```python
from build123d import *

# Parameters (mm, degrees)
SKETCH_1_W          = 8
SKETCH_1_H          = 29.75
SKETCH_1_R          = 1.5
EXTRUDE_1_DEPTH     = 1.5
SKETCH_2_W          = 2
SKETCH_2_H          = 8
EXTRUDE_2_DEPTH     = 16.5
FILLET_1_R          = 1
FILLET_2_R          = 1
SKETCH_4_R          = 1.5
CUT_EXTRUDE_1_DEPTH = 2


with BuildPart() as part:
    # 草图1 → 凸台-拉伸1 (new body)
    with BuildSketch(Plane.XY):
        Rectangle(SKETCH_1_W, SKETCH_1_H)
        with Locations((0, 11.875)):
            Circle(SKETCH_1_R, mode=Mode.SUBTRACT)
        with Locations((0, -11.875)):
            Circle(SKETCH_1_R, mode=Mode.SUBTRACT)
    extrude(amount=EXTRUDE_1_DEPTH)

    # 草图2 → 凸台-拉伸2 (add)
    with BuildSketch(Plane.XY.offset(1.5)):
        with Locations((0, 5)):
            Rectangle(SKETCH_2_W, SKETCH_2_H)
    extrude(amount=EXTRUDE_2_DEPTH)

    # 圆角1
    fillet_1_edges = [part.edges().sort_by_distance(p)[0] for p in [
        (1, 5, 1.5),
        (-1, 5, 1.5),
    ]]
    fillet(fillet_1_edges, radius=FILLET_1_R)

    # 圆角2
    fillet_2_edges = [part.edges().sort_by_distance(p)[0] for p in [
        (0, 9, 18),
        (0, 1, 18),
        (4, -14.875, 0.75),
        (-4, -14.875, 0.75),
        (-4, 14.875, 0.75),
        (4, 14.875, 0.75),
    ]]
    fillet(fillet_2_edges, radius=FILLET_2_R)

    # 草图4 → 切除-拉伸1 (cut)
    with BuildSketch(Plane.ZY.offset(1)):
        with Locations((14, 5)):
            Circle(SKETCH_4_R)
    extrude(amount=-CUT_EXTRUDE_1_DEPTH, mode=Mode.SUBTRACT)


solid = part.part
```
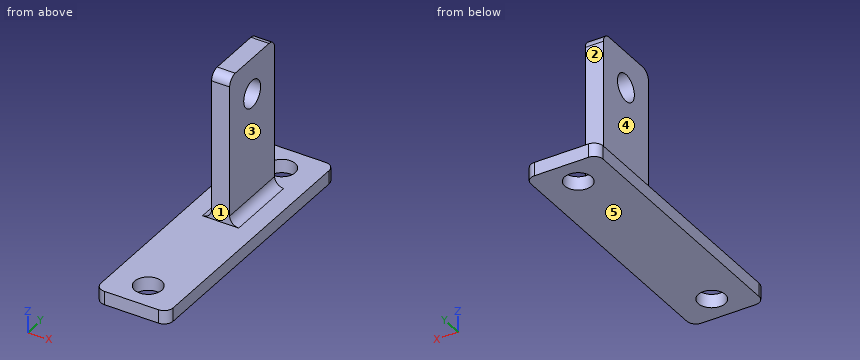
Verification items for the finished model (mm, model axes). Face numbers are marked on the shaded views. A direction names the side the tool comes from. Coordinates: 2 decimals unless noted, no trailing zeros. Write each loop counter-clockwise with the first axis right and the second up, starting at its lowest first coordinate (ties: lowest second). Pieces come first, ordered by that corner, then holes. Notation, with made-up numbers: (14.5, -2) - (72.5, -2) arc R13 cw to (72.5, 8) - close; hole circle Ø11 at (10.5, -14.75). An arc over 180 degrees is marked (long way). One line per question, with ' | ' between items. Start each with the question number.
1. Material ranges on line 1 along Y through (x, z) = (0, 1.25) (3 decimals); line 2 along Y through (x, z) = (-0.25, 14); line 3 along Z through (x, y) = (2, 9.5), recorded low to high.
2. Section check D-D (x = -2.5). Enter the section's corners in (y, z) (3 decimals).
3. Gauge pin test, flat ends, axial feed: P1, Ø8, axis at y = 0, z = 13, coming from the -X side; P2, Ø1.8, axis at x = 0, y = -11.875, coming from the -Z side; P3, Ø1.2, axis at x = 0.5, z = 10, coming from the -Y side; P4, Ø3, axis at x = -0.5, y = -5.5, coming from the +Z side. Record the tip position at first contact, or that the pin passes through.
4. Section check A-A (y = 5). Enter the section's corners in (x, z), plus the area to 3 significant figures.
5. Access from +Z, -Z, +X, -X, +Y, -Y to the whole of each face (thin tool, end or side, straight path). Record for the marked faces 1, 2, 3, 4 and 5.
6. Section check C-C (z = 14). Enter the section's corners in (x, y).
7. Section check B-B (x = 0). Enter the section's corners in (y, z) (3 decimals), plus the area to 3 significant figures.
Computed values:
1) line 1: -14.875 to -13.375, -10.375 to 10.375, 13.375 to 14.875 | line 2: 1 to 3.5, 6.5 to 9 | line 3: 0 to 1.5
2) outline: (-14.875, 0) - (14.875, 0) - (14.875, 1.5) - (-14.875, 1.5) - close
3) P1: x = -1 | P2: through | P3: y = 1 | P4: z = 1.5
4) outline: (-4, 0) - (4, 0) - (4, 1.5) - (2, 1.5) arc R1 cw to (1, 2.5) - (1, 12.5) - (-1, 12.5) - (-1, 2.5) arc R1 cw to (-2, 1.5) - (-4, 1.5) - close; (-1, 15.5) - (1, 15.5) - (1, 18) - (-1, 18) - close | area: 39.4 mm²
5) face 1: +Z, +X, -X, -Y | face 2: +Z, +X, -X, +Y | face 3: +Z, +X, +Y, -Y | face 4: +Z, -X, +Y, -Y | face 5: -Z, +X, -X, +Y, -Y
6) outline: (-1, 1) - (1, 1) - (1, 3.5) - (-1, 3.5) - close; (-1, 6.5) - (1, 6.5) - (1, 9) - (-1, 9) - close
7) outline: (-14.875, 0) - (-13.375, 0) - (-13.375, 1.5) - (-14.875, 1.5) - close; (-10.375, 0) - (10.375, 0) - (10.375, 1.5) - (9, 1.5) - (9, 17) arc R1 ccw to (8, 18) - (2, 18) arc R1 ccw to (1, 17) - (1, 1.5) - (-10.375, 1.5) - close; (13.375, 0) - (14.875, 0) - (14.875, 1.5) - (13.375, 1.5) - close; hole circle Ø3 at (5, 14) | area: 160 mm²
